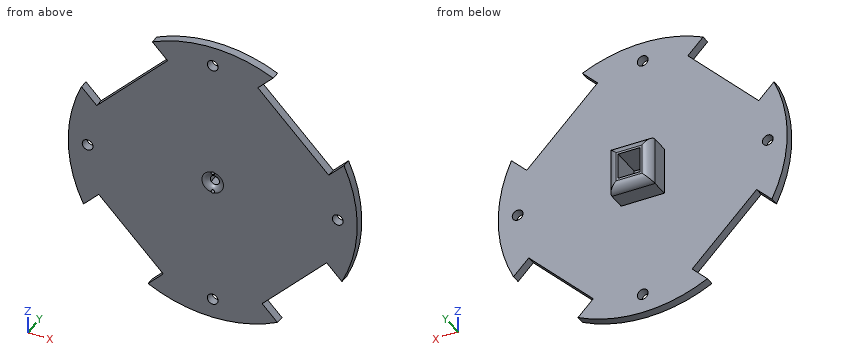
from build123d import *

# Parameters (mm, degrees)
SKETCH1_R           = 67
SKETCH1_R_2         = 2.5
BOSS_EXTRUDE1_DEPTH = 4
SKETCH2_R           = 2
CUT_EXTRUDE1_DEPTH  = 4
SKETCH4_W           = 20
SKETCH4_H           = 22
SKETCH4_W_2         = 10
SKETCH4_H_2         = 12
BOSS_EXTRUDE2_DEPTH = 12
FILLET1_R           = 4
FILLET2_R           = 3
CUT_EXTRUDE2_START  = -10
CUT_EXTRUDE2_DEPTH  = 10
SKETCH7_R           = 0.75
CUT_EXTRUDE3_DEPTH  = 10
SKETCH8_W           = 10
SKETCH8_H           = 12
CUT_EXTRUDE4_DEPTH  = 2


with BuildPart() as part:
    # Sketch1 → Boss-Extrude1 (new body)
    with BuildSketch(Plane(origin=(0, 0, 0), x_dir=(1, 0, 0), z_dir=(0, 1, 0))):
        with Locations(Location((0, 0, 0), (0, 0, 270))):
            Circle(SKETCH1_R)
        with Locations(Location((-58, 0, 0), (0, 0, 270))):
            Circle(SKETCH1_R_2, mode=Mode.SUBTRACT)
        with Locations(Location((0, -58, 0), (0, 0, 270))):
            Circle(SKETCH1_R_2, mode=Mode.SUBTRACT)
        with Locations(Location((58, 0, 0), (0, 0, 270))):
            Circle(SKETCH1_R_2, mode=Mode.SUBTRACT)
        with Locations(Location((0, 58, 0), (0, 0, 270))):
            Circle(SKETCH1_R_2, mode=Mode.SUBTRACT)
    extrude(amount=BOSS_EXTRUDE1_DEPTH)

    # Sketch2 → Cut-Extrude1 (cut)
    with BuildSketch(Plane(origin=(0, 4, 0), x_dir=(1, 0, 0), z_dir=(0, 1, 0))):
        with Locations(Location((0, 0, 0), (0, 0, 270))):
            Circle(SKETCH2_R)
    extrude(amount=-CUT_EXTRUDE1_DEPTH, mode=Mode.SUBTRACT)

    # Sketch4 → Boss-Extrude2 (add)
    with BuildSketch(Plane(origin=(0, 4, 0), x_dir=(1, 0, 0), z_dir=(0, 1, 0))):
        Rectangle(SKETCH4_W, SKETCH4_H)
        Rectangle(SKETCH4_W_2, SKETCH4_H_2, mode=Mode.SUBTRACT)
    extrude(amount=BOSS_EXTRUDE2_DEPTH)

    # Fillet1
    fillet1_edges = [part.edges().sort_by_distance(p)[0] for p in [
        (10, 16, 0),
        (0, 16, -11),
        (-10, 16, 0),
        (0, 16, 11),
    ]]
    fillet(fillet1_edges, radius=FILLET1_R)

    # Fillet2
    fillet2_edges = [part.edges().sort_by_distance(p)[0] for p in [
        (0, 0, -2),
    ]]
    fillet(fillet2_edges, radius=FILLET2_R)

    # Sketch5 → Cut-Extrude2 (cut)
    with BuildSketch(Plane(origin=(0, 4, 0), x_dir=(1, 0, 0), z_dir=(0, 1, 0)).offset(CUT_EXTRUDE2_START)):
        with BuildLine():
            Line((59.908263203, 30), (52.837195391, 22.928932188))
            Line((52.837195391, 22.928932188), (22.928932188, 52.837195391))
            Line((22.928932188, 52.837195391), (30, 59.908263203))
            ThreePointArc((30, 59.908263203), (47.376154339, 47.376154339), (59.908263203, 30))
        make_face()
        with BuildLine():
            Line((-59.908263203, 30), (-52.837195391, 22.928932188))
            Line((-52.837195391, 22.928932188), (-22.928932188, 52.837195391))
            Line((-22.928932188, 52.837195391), (-30, 59.908263203))
            ThreePointArc((-30, 59.908263203), (-47.376154339, 47.376154339), (-59.908263203, 30))
        make_face()
        with BuildLine():
            Line((-53.797643362, -20.928932188), (-20.928932188, -53.797643362))
            Line((-20.928932188, -53.797643362), (-28, -60.868711174))
            ThreePointArc((-28, -60.868711174), (-47.376154339, -47.376154339), (-60.868711174, -28))
            Line((-60.868711174, -28), (-53.797643362, -20.928932188))
        make_face()
        with BuildLine():
            Line((53.797643362, -20.928932188), (20.928932188, -53.797643362))
            Line((20.928932188, -53.797643362), (28, -60.868711174))
            ThreePointArc((28, -60.868711174), (47.376154339, -47.376154339), (60.868711174, -28))
            Line((60.868711174, -28), (53.797643362, -20.928932188))
        make_face()
    extrude(amount=CUT_EXTRUDE2_DEPTH, mode=Mode.SUBTRACT)

    # Sketch7 → Cut-Extrude3 (cut)
    with BuildSketch(Plane(origin=(0, 4, 0), x_dir=(1, 0, 0), z_dir=(0, 1, 0))):
        with Locations(Location((0, 4.5, 0), (0, 0, 270))):
            Circle(SKETCH7_R)
        with Locations(Location((0, -4.5, 0), (0, 0, 270))):
            Circle(SKETCH7_R)
    extrude(amount=-CUT_EXTRUDE3_DEPTH, mode=Mode.SUBTRACT)

    # Sketch8 → Cut-Extrude4 (cut)
    with BuildSketch(Plane(origin=(0, 4, 0), x_dir=(1, 0, 0), z_dir=(0, 1, 0))):
        Rectangle(SKETCH8_W, SKETCH8_H)
    extrude(amount=-CUT_EXTRUDE4_DEPTH, mode=Mode.SUBTRACT)


solid = part.part
CAD build for the part. Positions are in the model's coordinates, mm. Round coordinates to 2 decimals unless told otherwise and drop trailing zeros. Loops run counter-clockwise (first coordinate to the right, second up) from the corner with the lowest first, then second, coordinate; pieces in that order, holes last.
(1) Drop flat-ended pins along their axis: pin 1 (6.5 mm diameter, centred on y = 7, z = -2.5, fed in from -X); pin 2 (4 mm diameter, centred on y = 9.5, z = -2, fed in from +X); pin 3 (6.5 mm diameter, centred on x = 4, y = 6, fed in from -Z). Give the stop position or say it passes through.
(2) Wall check: line 1 along Y through (x, z) = (50.5, -23); line 2 along X through (y, z) = (0.6, -4.5); line 3 along X through (y, z) = (1.05, 0). Give the ranges that are in metal, low to high.
(3) Cut at D-D (z = -27.5). Give the cut face in (x, y), plus the area to 3 significant figures.
(4) Cut at C-C (x = -58). Give the cut face in (y, z), plus the area to 3 significant figures.
(5) Cut at A-A (y = 7). Give the cut face in (x, z).
(6) Cut at B-B (z = -57.5). Give the cut face in (x, y).
Findings below:
1. pin 1: stops at x = -66.99
1. pin 2: stops at x = 10
1. pin 3: stops at z = -66.98
2. line 1: y = 0 to 4
2. line 2: x = -66.85 to -0.75, 0.75 to 66.85
2. line 3: x = -67 to -60.5, -55.5 to -2.72, 2.72 to 55.5, 60.5 to 67
3. outline: (-61.1, 0) - (-57.41, 0) - (-57.41, 4) - (-61.1, 4) - close; (-48.27, 0) - (48.27, 0) - (48.27, 4) - (-48.27, 4) - close; (57.41, 0) - (61.1, 0) - (61.1, 4) - (57.41, 4) - close
3. area: 416 mm2
4. outline: (0, -28.09) - (4, -28.09) - (4, -2.5) - (0, -2.5) - close; (0, 2.5) - (4, 2.5) - (4, 25.13) - (0, 25.13) - close
4. area: 193 mm2
5. outline: (-10, -11) - (10, -11) - (10, 11) - (-10, 11) - close; hole (-5, -6) - (5, -6) - (5, 6) - (-5, 6) - close
6. outline: (-27.59, 0) - (-2.45, 0) - (-2.45, 4) - (-27.59, 4) - close; (2.45, 0) - (27.59, 0) - (27.59, 4) - (2.45, 4) - close
